Print and shaded views of the part. All mm, measured from the part's lowest x, y and z. Round coordinates to 2 decimals unless told otherwise and drop trailing zeros. Loops run counter-clockwise (first coordinate to the right, second up) from the corner with the lowest first, then second, coordinate; pieces in that order, holes last. Notation, with made-up numbers: (-25.75, -29.75) - (31.25, -29.75) arc R22 ccw to (31.25, -15.75) - close; hole circle Ø10 at (33, 43). An arc over 180 degrees is marked (long way). Use one line per item in the form item = value. Start each with the question number.
Q1. Saw through at A-A (x = 86.5). Give the cut face in (y, z), then the cut area to 3 significant figures.
Q2. Saw through at D-D (x = 13.5). Give the cut face in (y, z), then the cut area to 3 significant figures.
Q3. Saw through at C-C (y = 11). Give the cut face in (x, z).
Q4. Drill centre lines: line 1 (X direction, y = 0.5, z = 79); line 2 (Y direction, x = 101, z = 69.5); line 3 (Y direction, x = 29, z = 68). Where is each one in solid material? Low to high.
Q5. Pin check, flat tips, straight feed: pin 1 (1 mm diameter, centred on x = 59, z = 91.5, fed in from -Y); pin 2 (6 mm diameter, centred on x = 83.5, y = 10, fed in from +Z); pin 3 (4 mm diameter, centred on x = 49.5, z = 30, fed in from +Y). Stop position of each tip, or through.
Q6. Mould opens along X. For the marked faces 1 and 2 say: released by +X, released by -X, zero draft, split by the parting line, or undercut.
Q7. Saw through at B-B (z = 60). Give the cut face in (x, y), then the cut area to 3 significant figures.
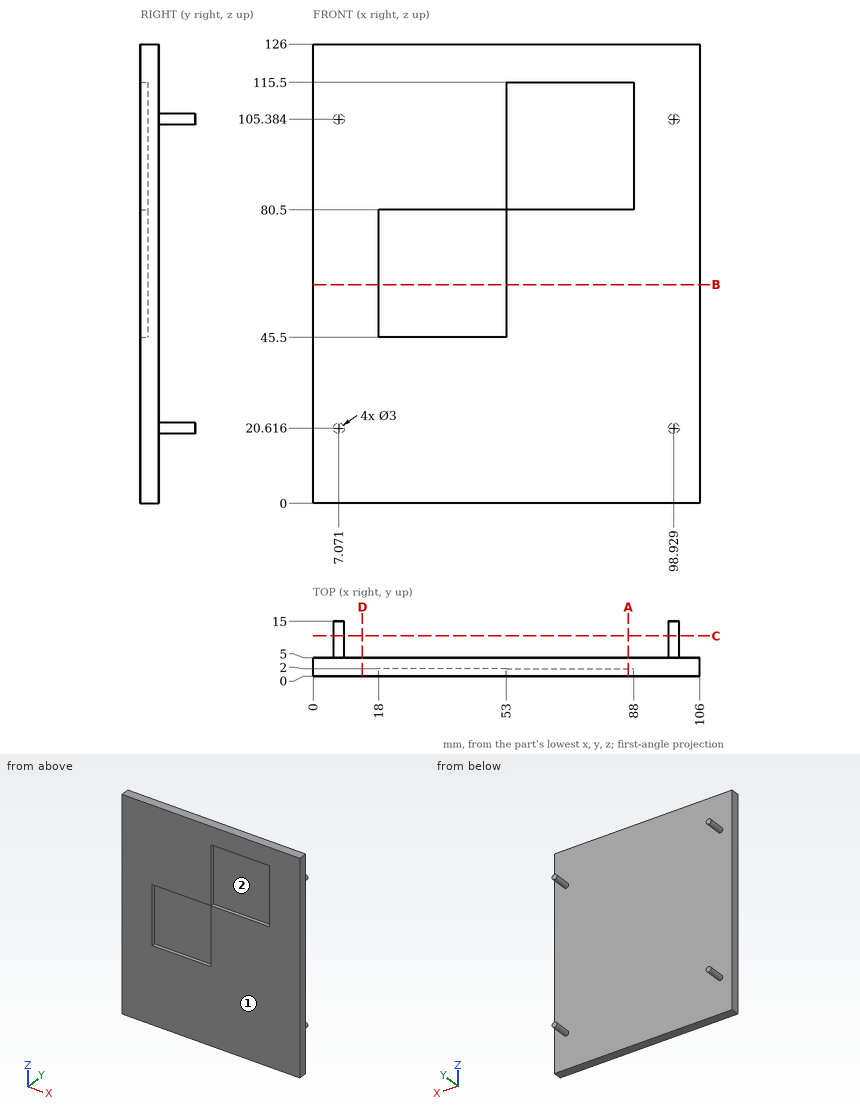
Report:
q1.outline = (0, 0) - (5, 0) - (5, 126) - (0, 126) - (0, 115.5) - (2, 115.5) - (2, 80.5) - (0, 80.5) - close
q1.area = 560 mm²
q2.outline = (0, 0) - (5, 0) - (5, 126) - (0, 126) - close
q2.area = 630 mm²
q3.outline = circle Ø3 at (7.07, 20.62); circle Ø3 at (7.07, 105.38); circle Ø3 at (98.93, 20.62); circle Ø3 at (98.93, 105.38)
q4.line_1 = 0 to 18, 53 to 106
q4.line_2 = 0 to 5
q4.line_3 = 2 to 5
q5.pin_1 = 2
q5.pin_2 = through
q5.pin_3 = 5
q6.face_1 = zero draft
q6.face_2 = undercut
q7.outline = (0, 0) - (18, 0) - (18, 2) - (53, 2) - (53, 0) - (106, 0) - (106, 5) - (0, 5) - close
q7.area = 460 mm²
